Input: part model. Units: mm. Frame: model coordinates. A direction names the side the tool comes from. Give positions to 0.01 mm unless a question says otherwise; leave off trailing zeros. Loops run counter-clockwise (first coordinate to the right, second up) from the corner with the lowest first, then second, coordinate; pieces in that order, holes last.
from build123d import *

# Parameters (mm, degrees)
SKETCH1_R                      = 7.5
SKETCH1_R_2                    = 4
BOSS_EXTRUDE1_DEPTH            = 32
SKETCH6_W                      = 1
SKETCH6_H                      = 1
SKETCH7_W                      = 1
SKETCH7_H                      = 1
CUT_EXTRUDE1_DEPTH             = 35.18332927
BOSS_EXTRUDE3_DEPTH            = 6.5
SKETCH15_W                     = 15.5
SKETCH15_H                     = 12.485281374
CUT_EXTRUDE2_DEPTH             = 0.5
CBORE_FOR_M2_SHCS1_D           = 2.2
CBORE_FOR_M2_SHCS1_CBORE_D     = 4.4
CBORE_FOR_M2_SHCS1_CBORE_DEPTH = 4
FILLET4_R                      = 0.5
SKETCH4_R                      = 7.75
SKETCH4_R_2                    = 4
BOSS_EXTRUDE4_DEPTH            = 1
CUT_EXTRUDE3_DEPTH             = 4
FILLET5_R                      = 1


with BuildPart() as part:
    # Sketch1 → Boss-Extrude1 (new body)
    with BuildSketch(Plane.XY):
        Circle(SKETCH1_R)
        Circle(SKETCH1_R_2, mode=Mode.SUBTRACT)
    extrude(amount=BOSS_EXTRUDE1_DEPTH)

    # Sketch6 → Revolve1 (revolve)
    with BuildSketch(Plane(origin=(0, 0, 0), x_dir=(-1, 0, 0), z_dir=(0, 1, 0))):
        with Locations((8, 0.5)):
            Rectangle(SKETCH6_W, SKETCH6_H)
    revolve(axis=Axis((0, 0, 32), (0, 0, -1)))

    # Sketch7 → Revolve2 (revolve)
    with BuildSketch(Plane(origin=(0, 0, 0), x_dir=(0, 0, -1), z_dir=(1, 0, 0)), mode=Mode.PRIVATE) as revolve2_sk:
        with Locations((-7, 8)):
            Rectangle(SKETCH7_W, SKETCH7_H)
    revolve(revolve2_sk.sketch.rotate(Axis((0, 0, 32), (0, 0, -1)), 270), axis=Axis((0, 0, 32), (0, 0, -1)))

    # Sketch9 → Cut-Extrude1 (cut, through all)
    with BuildSketch(Plane(origin=(0, 0, 0), x_dir=(-1, 0, 0), z_dir=(0, 1, 0))):
        Polygon((0, 0), (-0.5, 0), (-0.5, 6.5), (0.5, 6.5), (0.5, 0), align=None)
    extrude(amount=CUT_EXTRUDE1_DEPTH, mode=Mode.SUBTRACT)

    # Sketch12 → Boss-Extrude3 (add)
    with BuildSketch(Plane(origin=(0, 0, 6.5), x_dir=(-1, 0, 0), z_dir=(0, 0, -1))):
        with BuildLine():
            Line((4, 0), (7.75, 0))
            Line((7.75, 0), (7.75, 8.485281374))
            Line((7.75, 8.485281374), (0.5, 8.485281374))
            Line((0.5, 8.485281374), (0.5, 3.968626967))
            ThreePointArc((0.5, 3.968626967), (3, 2.645751311), (4, 0))
        make_face()
        with BuildLine():
            Line((-7.75, 0), (-7.75, 8.485281374))
            Line((-7.75, 8.485281374), (-0.5, 8.485281374))
            Line((-0.5, 8.485281374), (-0.5, 3.968626967))
            ThreePointArc((-0.5, 3.968626967), (-3, 2.645751311), (-4, 0))
            Line((-4, 0), (-7.75, 0))
        make_face()
    extrude(amount=BOSS_EXTRUDE3_DEPTH)

    # Sketch15 → Cut-Extrude2 (cut)
    with BuildSketch(Plane(origin=(0, 0, 6.5), x_dir=(-1, 0, 0), z_dir=(0, 0, -1))):
        with Locations((0, 2.242640687)):
            Rectangle(SKETCH15_W, SKETCH15_H)
    extrude(amount=CUT_EXTRUDE2_DEPTH, mode=Mode.SUBTRACT)

    # CBORE for M2 SHCS1 (through all)
    with Locations(Plane(origin=(-7.75, 5.988170693, 3), x_dir=(0, 0, -1), z_dir=(-1, 0, 0))):
        with Locations((0, 0)):
            CounterBoreHole(CBORE_FOR_M2_SHCS1_D / 2, CBORE_FOR_M2_SHCS1_CBORE_D / 2, CBORE_FOR_M2_SHCS1_CBORE_DEPTH)

    # Fillet4
    fillet4_edges = [part.edges().sort_by_distance(p)[0] for p in [
        (-6.34428877, -4, 6.25),
        (6.34428877, -4, 6.25),
    ]]
    fillet(fillet4_edges, radius=FILLET4_R)

    # Sketch4 → Boss-Extrude4 (add)
    with BuildSketch(Plane.XY.offset(29)):
        Circle(SKETCH4_R)
        with Locations(Location((0, 0, 0), (0, 0, 270))):
            Circle(SKETCH4_R_2, mode=Mode.SUBTRACT)
    extrude(amount=BOSS_EXTRUDE4_DEPTH)

    # Sketch16 → Cut-Extrude3 (cut)
    with BuildSketch(Plane(origin=(7.75, 0, 0), x_dir=(0, 0, -1), z_dir=(1, 0, 0))):
        Polygon((-3, 8.297571769), (-5, 7.142871231), (-5, 4.833470154), (-3, 3.678769616), (-1, 4.833470154), (-1, 7.142871231), align=None)
    extrude(amount=-CUT_EXTRUDE3_DEPTH, mode=Mode.SUBTRACT)

    # Fillet5
    # the kernel refuses this fillet: 1 mm, written as the material it takes off along each edge
    with BuildSketch(Plane(origin=(0.5, 8.485281374, 6), x_dir=(0, -1, 0), z_dir=(0, 0, -1))) as fillet5_piece_1:
        with BuildLine():
            CenterArc((FILLET5_R, -FILLET5_R), FILLET5_R, 90, 90)
            Line((0, -FILLET5_R), (0, 0))
            Line((0, 0), (FILLET5_R, 0))
        make_face()
    extrude(amount=8.5, mode=Mode.SUBTRACT)
    with BuildSketch(Plane(origin=(-2, 8.485281374, 6), x_dir=(0, -1, 0), z_dir=(1, 0, 0)), Plane(origin=(-10.25, 8.485281374, 6), x_dir=(0, -1, 0), z_dir=(1, 0, 0)), Plane(origin=(-10.25, 8.485281374, 0), x_dir=(0, 0, 1), z_dir=(1, 0, 0))) as fillet5_piece_2:
        with BuildLine():
            CenterArc((FILLET5_R, FILLET5_R), FILLET5_R, 180, 90)
            Line((0, FILLET5_R), (0, 0))
            Line((0, 0), (FILLET5_R, 0))
        make_face()
    extrude(amount=12.25, mode=Mode.SUBTRACT)
    with BuildSketch(Plane(origin=(0, 0, 0), x_dir=(0.0031415874858760906, 0.9999950652018582, 0), z_dir=(-0.9999950652018582, 0.0031415874858760906, 0))) as fillet5_piece_3:
        with BuildLine():
            CenterArc((4 + FILLET5_R, -FILLET5_R), FILLET5_R, 90, 90)
            Line((4 + FILLET5_R, 0), (4, 0))
            Line((4, 0), (4, -FILLET5_R))
        make_face()
    revolve(axis=Axis((0, 0, 0), (0, 0, -1)), revolution_arc=359.64, mode=Mode.SUBTRACT)
    with BuildSketch(Plane(origin=(-0.5, 8.485281374, -2.5), x_dir=(-1, 0, 0), z_dir=(0, 0, 1))) as fillet5_piece_4:
        with BuildLine():
            CenterArc((FILLET5_R, FILLET5_R), FILLET5_R, 180, 90)
            Line((0, FILLET5_R), (0, 0))
            Line((0, 0), (FILLET5_R, 0))
        make_face()
    extrude(amount=8.5, mode=Mode.SUBTRACT)
    with BuildSketch(Plane(origin=(0, 0, 32), x_dir=(1, 0, 0), z_dir=(0, -1, 0))) as fillet5_piece_5:
        with BuildLine():
            CenterArc((4 + FILLET5_R, -FILLET5_R), FILLET5_R, 90, 90)
            Line((4 + FILLET5_R, 0), (4, 0))
            Line((4, 0), (4, -FILLET5_R))
        make_face()
    revolve(axis=Axis((0, 0, 32), (0, 0, 1)), mode=Mode.SUBTRACT)
    with BuildSketch(Plane(origin=(-7.75, 8.485281374, 8.5), x_dir=(0, -1, 0), z_dir=(0, 0, -1)), Plane(origin=(7.75, 8.485281374, 8.5), x_dir=(-1, 0, 0), z_dir=(0, 0, -1))) as fillet5_piece_6:
        with BuildLine():
            CenterArc((FILLET5_R, -FILLET5_R), FILLET5_R, 90, 90)
            Line((0, -FILLET5_R), (0, 0))
            Line((0, 0), (FILLET5_R, 0))
        make_face()
    extrude(amount=11, mode=Mode.SUBTRACT)
    with BuildSketch(Plane(origin=(10.25, 8.485281374, 0), x_dir=(0, 0, 1), z_dir=(-1, 0, 0))) as fillet5_piece_7:
        with BuildLine():
            CenterArc((FILLET5_R, -FILLET5_R), FILLET5_R, 90, 90)
            Line((0, -FILLET5_R), (0, 0))
            Line((0, 0), (FILLET5_R, 0))
        make_face()
    extrude(amount=12.25, mode=Mode.SUBTRACT)


solid = part.part
(1) Cut plane A-A (z = 8.5). Return the cut outline in (x, y), and give its area (3 significant figures).
Values follow:
outline: circle Ø15 at (0, 0); hole circle Ø8 at (0, 0)
area: 126 mm2
(2) Mould query, pull axis X, two halves, no side actions, for faces 4 (the flat face through (0, -8, 1)), 5 (the cylindrical face through (0.237, -8.497, 0.507)), 6 (the cylindrical face through (-0.867, -3.905, 18.578)). Classes: +X half, -X half, draft (parallel to the pull), parting line (faces both ways), or undercut.
Values follow:
face 4: draft
face 5: parting line
face 6: undercut
(3) Cut plane D-D (y = -6). Return the cut outline in (x, z).
Values follow:
outline: (-6.02, 0) - (6.02, 0) - (6.02, 1) - (4.5, 1) - (4.5, 6.5) - (6.02, 6.5) - (6.02, 7.5) - (4.5, 7.5) - (4.5, 29) - (4.91, 29) - (4.91, 30) - (4.5, 30) - (4.5, 32) - (-4.5, 32) - (-4.5, 30) - (-4.91, 30) - (-4.91, 29) - (-4.5, 29) - (-4.5, 7.5) - (-6.02, 7.5) - (-6.02, 6.5) - (-4.5, 6.5) - (-4.5, 1) - (-6.02, 1) - close
(4) Pin query (flat end, axial travel): pin 1 Ø4 at (y, z) = (6.5, 3.5) entering from -X; pin 2 Ø1.2 at (x, z) = (3.5, 3.5) entering from +Y; pin 3 Ø5 at (x, z) = (-4, 25) entering from +Y. Return the tip coordinate at first contact, or that it passes through.
Values follow:
pin 1: stops at x = -7.75
pin 2: stops at y = 8.49
pin 3: stops at y = 7.35
(5) Cut plane B-B (x = -2). Count the separate pieces of the cut face and the enclosed holes in it, and give its area (3 significant figures).
Values follow:
separate pieces: 3
enclosed holes: 1
area: 245 mm2
(6) Ray query, probe 1 along Y at (x, z) = (0, 14); probe 2 along Z at (x, y) = (4.5, 6.75); probe 3 along Z at (x, y) = (-7, -4.5). Return the intervals inside material, ascending.
Values follow:
probe 1: y = -7.5 to -4, 4 to 7.5
probe 2: z = 0 to 1, 5 to 6, 6.5 to 7.5
probe 3: z = 0 to 1, 6.5 to 7.5
(7) Reachability of faces 1 (the cylindrical face through (-7.493, 0.33, 18.1)), 2 (the flat face through (-3.75, 5, 4)), 3 (the flat face through (5.78, 4.26, 4.01)) from +Z, -Z, +X, -X, +Y, -Y: full face, straight path, thin tool, end or side. Return the list, or none.
Values follow:
face 1: none
face 2: -X
face 3: +X
